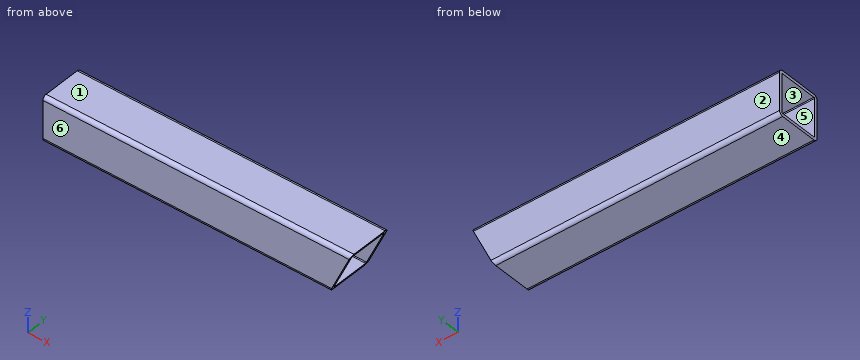
from build123d import *

# Parameters (mm, degrees)
EXTRUDE_THIN1_DEPTH     = 130.175
CUT_EXTRUDE1_DEPTH      = 1
CUT_EXTRUDE1_DEPTH_BACK = 39.1


with BuildPart() as part:
    # Sketch1 → Extrude-Thin1 (new body, symmetric)
    with BuildSketch(Plane(origin=(0, 0, 0), x_dir=(0, 0, -1), z_dir=(1, 0, 0))):
        with BuildLine():
            Line((-15.875, 19.05), (15.875, 19.05))
            ThreePointArc((15.875, 19.05), (18.12006403, 18.12006403), (19.05, 15.875))
            Line((19.05, 15.875), (19.05, -15.875))
            ThreePointArc((19.05, -15.875), (18.12006403, -18.12006403), (15.875, -19.05))
            Line((15.875, -19.05), (-15.875, -19.05))
            ThreePointArc((-15.875, -19.05), (-18.12006403, -18.12006403), (-19.05, -15.875))
            Line((-19.05, -15.875), (-19.05, 15.875))
            ThreePointArc((-19.05, 15.875), (-18.12006403, 18.12006403), (-15.875, 19.05))
        make_face()
        with BuildLine():
            Line((-15.875, 16.51), (15.875, 16.51))
            ThreePointArc((15.875, 16.51), (16.324012806, 16.324012806), (16.51, 15.875))
            Line((16.51, 15.875), (16.51, -15.875))
            ThreePointArc((16.51, -15.875), (16.324012806, -16.324012806), (15.875, -16.51))
            Line((15.875, -16.51), (-15.875, -16.51))
            ThreePointArc((-15.875, -16.51), (-16.324012806, -16.324012806), (-16.51, -15.875))
            Line((-16.51, -15.875), (-16.51, 15.875))
            ThreePointArc((-16.51, 15.875), (-16.324012806, 16.324012806), (-15.875, 16.51))
        make_face(mode=Mode.SUBTRACT)
    extrude(amount=EXTRUDE_THIN1_DEPTH, both=True)

    # Sketch3 → Cut-Extrude1 (cut, two sides)
    with BuildSketch(Plane(origin=(0, 19.05, 0), x_dir=(1, 0, 0), z_dir=(0, 1, 0))) as cut_extrude1_sk:
        Polygon((356.802383498, -505.053992289), (130.175, -19.05), (112.408678224, 19.05), (-114.218705274, 505.053992289), (857.789279304, 958.308759286), (1328.810368077, -51.799225292), align=None)
    extrude(amount=CUT_EXTRUDE1_DEPTH, mode=Mode.SUBTRACT)
    extrude(cut_extrude1_sk.sketch, amount=-CUT_EXTRUDE1_DEPTH_BACK, mode=Mode.SUBTRACT)


solid = part.part
Build history of the part. All positions in model axes, mm. Face numbers are marked on the shaded views. A direction names the side the tool comes from. Give positions to 0.01 mm unless a question says otherwise; leave off trailing zeros. Write each loop counter-clockwise with the first axis right and the second up, starting at its lowest first coordinate (ties: lowest second). Pieces come first, ordered by that corner, then holes. Notation, with made-up numbers: (29.5, 35.25) - (59.5, 35.25) arc R10 ccw to (59.5, 48.25) - close; hole circle Ø7 at (43, 51). An arc over 180 degrees is marked (long way). Use one line per item in the form item = value. Start each with the question number.
1. Band-saw the part on B-B on z = 4.5. Write the cut outline in (x, y) (3 decimals), plus the area to 3 significant figures.
2. Band-saw the part on C-C on x = -9. Write the cut outline in (y, z) (3 decimals).
3. Probe line 1 (Y direction, x = -111, z = 0); line 2 (X direction, y = 15, z = 17) (3 decimals). List the from-to ranges inside material, lowest first. Write a range as [from, to].
4. Drop a flat-ended pin along its axis: pin 1 Ø6 at (y, z) = (13, -3.5) entering from +X. Give the stop position or say it passes through.
5. Band-saw the part on A-A on y = -5. Write the cut outline in (x, z) (3 decimals), plus the area to 3 significant figures.
6. 3-axis set-ups, long thin cutter, end or side, ignore diameter. For the marked faces 5 and 6: which of +Z, -Z, +X, -X, +Y, -Y reach the whole face in a straight line?
7. Two-plate mould, pull along Z, no slides. Class the marked faces 1, 2, 3 and 4: released by +Z, released by -Z, zero draft, split by the parting line, or undercut.
Conclusion:
q1.outline = (-130.175, -19.05) - (123.39, -19.05) - (123.39, -16.51) - (-130.175, -16.51) - close; (-130.175, 16.51) - (123.39, 16.51) - (123.39, 19.05) - (-130.175, 19.05) - close
q1.area = 1,290 mm²
q2.outline = (-19.05, -15.875) arc R3.175 ccw to (-15.875, -19.05) - (15.875, -19.05) arc R3.175 ccw to (19.05, -15.875) - (19.05, 15.875) arc R3.175 ccw to (15.875, 19.05) - (-15.875, 19.05) arc R3.175 ccw to (-19.05, 15.875) - close; hole (-16.51, -15.875) arc R0.635 ccw to (-15.875, -16.51) - (15.875, -16.51) arc R0.635 ccw to (16.51, -15.875) - (16.51, 15.875) arc R0.635 ccw to (15.875, 16.51) - (-15.875, 16.51) arc R0.635 ccw to (-16.51, 15.875) - close
q3.line_1 = [-19.05, -16.51], [16.51, 19.05]
q3.line_2 = [-130.175, 129.219]
q4.pin_1 = through
q5.outline = (-130.175, -19.05) - (112.409, -19.05) - (113.593, -16.51) - (-130.175, -16.51) - close; (-130.175, 16.51) - (128.991, 16.51) - (130.175, 19.05) - (-130.175, 19.05) - close
q5.area = 1,280 mm²
q6.face_5 = +X, -X
q6.face_6 = +Z, -Z, +X, -X, -Y
q7.face_1 = released by +Z
q7.face_2 = zero draft
q7.face_3 = undercut
q7.face_4 = released by -Z
